from build123d import *

# Parameters (mm, degrees)
F0_R     = 6.35
F0_R_2   = 23.01875
F1_DEPTH = 19.05
F2_SIZE  = 1.5875


with BuildPart() as f1:
    # F0 (on Top) → F1 (new body)
    with BuildSketch(Plane.XY):
        Polygon((-19.05, -31.75), (19.05, -31.75), (50.8, -12.7), (50.8, 12.7), (19.05, 31.75), (-19.05, 31.75), (-50.8, 12.7), (-50.8, -12.7), align=None)
        with Locations((-38.1, 0)):
            Circle(F0_R, mode=Mode.SUBTRACT)
        Circle(F0_R_2, mode=Mode.SUBTRACT)
        with Locations((38.1, 0)):
            Circle(F0_R, mode=Mode.SUBTRACT)
    extrude(amount=F1_DEPTH)

    # F2
    f2_edges = [f1.edges().sort_by_distance(p)[0] for p in [
        (-23.01875, 0, 0),
        (-23.01875, 0, 19.05),
    ]]
    chamfer(f2_edges, length=F2_SIZE)


solid = f1.part
Geometry: final body of the model. Coordinates: model frame, mm. Round coordinates to 2 decimals unless told otherwise and drop trailing zeros. Loops run counter-clockwise (first coordinate to the right, second up) from the corner with the lowest first, then second, coordinate; pieces in that order, holes last. Notation, with made-up numbers: M 41,58.5 L 64,58.5 A15 ccw 64,68.5 Z; hole C 80.5,66 d4. An arc over 180 degrees is marked long. One line per question, with ' | ' between items.
(1) Cut plane D-D on y = 3.5. Give the number of separate pieces and of enclosed holes in the cut face, plus the area to 3 significant figures.
Check result:
separate pieces: 4 | enclosed holes: 0 | area: 660 mm2
(2) Pull-direction query (Y, two-part tool) for faces 1 (the flat face through (-34.7, 22.36, 9.39)), 2 (the cylindrical face through (-32.043, 1.907, 9.392)), 3 (the flat face through (0, -31.75, 9)); classes: +Y half, -Y half, draft (parallel to the pull), parting line (faces both ways), or undercut.
Check result:
face 1: +Y half | face 2: undercut | face 3: -Y half
(3) Material intervals for line 1 along X through (y, z) = (17.5, 11); line 2 along X through (y, z) = (3.5, 17); line 3 along Y through (x, z) = (-42, 7), sorted ascending. Write a range as from..to.
Check result:
line 1: x = -42.8..-14.95, 14.95..42.8 | line 2: x = -50.8..-43.4, -32.8..-22.75, 22.75..32.8, 43.4..50.8 | line 3: y = -17.98..-5.01, 5.01..17.98
(4) Cut plane A-A on x = -38.1. Return the cut outline in (y, z), plus the area to 3 significant figures.
Check result:
outline: M -20.32,0 L -6.35,0 L -6.35,19.05 L -20.32,19.05 Z; M 6.35,0 L 20.32,0 L 20.32,19.05 L 6.35,19.05 Z | area: 532 mm2
(5) Cut plane C-C on x = 0. Return the cut outline in (y, z), plus the area to 3 significant figures.
Check result:
outline: M -31.75,0 L -24.61,0 L -23.02,1.59 L -23.02,17.46 L -24.61,19.05 L -31.75,19.05 Z; M 23.02,1.59 L 24.61,0 L 31.75,0 L 31.75,19.05 L 24.61,19.05 L 23.02,17.46 Z | area: 328 mm2
(6) Contact query for flat-ended pins moving along their axis: P1, Ø1, axis at x = -16, y = -13.5, coming from the -Z side; P2, Ø6, axis at x = 32.5, z = 2, coming from the -Y side; P3, Ø4, axis at x = 13, y = 18, coming from the +Z side; P4, Ø1, axis at x = -29.5, z = 11.5, coming from the -Y side. Output: stop coordinate, or through.
Check result:
P1: passes through | P2: stops at y = -25.48 | P3: stops at z = 18.65 | P4: stops at y = -25.78
(7) Cut plane B-B on z = 3.25. Return the cut outline in (x, y), plus the area to 3 significant figures.
Check result:
outline: M -50.8,-12.7 L -19.05,-31.75 L 19.05,-31.75 L 50.8,-12.7 L 50.8,12.7 L 19.05,31.75 L -19.05,31.75 L -50.8,12.7 Z; hole C -38.1,0 d12.7; hole C 0,0 d46.04; hole C 38.1,0 d12.7 | area: 3,320 mm2
